For this review, take the finished solid that the model builds, in its own axes (mm). Face numbers are marked on the shaded views. A direction names the side the tool comes from. Round coordinates to 2 decimals unless told otherwise and drop trailing zeros. Order: outer loops, then holes, each group sorted by start corner. A loop starts at its lowest first (then second) coordinate and runs counter-clockwise, first axis right, second up. Notation, with made-up numbers: M 36.5,65 L 85.5,65 A17 ccw 85.5,90 Z; hole C 16.5,7 d2. An arc over 180 degrees is marked long. Write item = value, one per line. Start each with the question number.
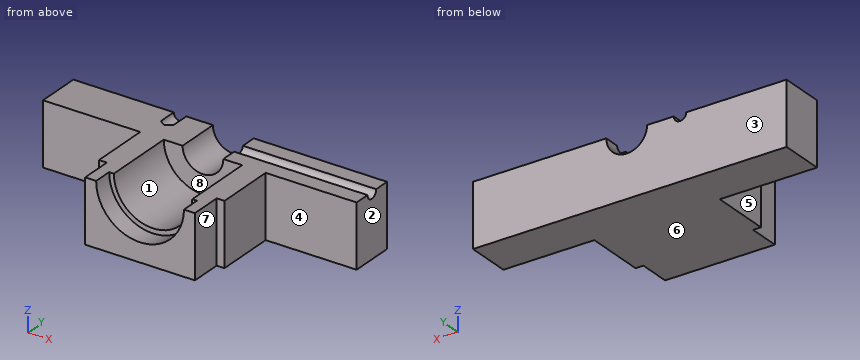
from build123d import *

# Parameters (mm, degrees)
PAD_DEPTH    = 20
SKETCH002_R  = 2
POCKET_DEPTH = 50


with BuildPart() as part:
    # Sketch → Pad (new body)
    with BuildSketch(Plane.XY):
        Polygon((-51, 0), (49, 0), (49, -14), (20, -14), (20, -33), (17.5, -33), (17.5, -43), (-17.5, -43), (-17.5, -33), (-20, -33), (-20, -14), (-51, -14), align=None)
    extrude(amount=-PAD_DEPTH)

    # Sketch001 → Groove (revolve, cut)
    with BuildSketch(Plane.XY):
        Polygon((0, 0), (6.5, 0), (6.5, -14), (12.5, -14), (12.5, -37), (14, -37), (14, -45), (0, -45), align=None)
    revolve(axis=Axis((0, 0, 0), (0, 1, 0)), mode=Mode.SUBTRACT)

    # Sketch002 → Pocket (cut)
    with BuildSketch(Plane.YZ):
        with Locations((-7, 0)):
            Circle(SKETCH002_R)
    extrude(amount=POCKET_DEPTH, mode=Mode.SUBTRACT)

    # Sketch003 → Groove001 (revolve, cut)
    with BuildSketch(Plane(origin=(-17, 0, 0), x_dir=(1, 0, 0), z_dir=(0, 0, 1))):
        Polygon((0, 0), (2, 0), (2, -6), (0, -7.201721), align=None)
    revolve(axis=Axis((-17, 0, 0), (0, 1, 0)), mode=Mode.SUBTRACT)


solid = part.part
(1) For line 1 along Y through (x, z) = (20.5, -4); line 2 along X through (y, z) = (-36.5, -17.5); line 3 along X through (y, z) = (-27, -10), list the stretches that pass through material, from the lowest coordinate up.
(2) Insertion check: pin 1 (8 mm diameter, centred on y = -39.5, z = -14.5, fed in from -X); pin 2 (6 mm diameter, centred on x = 32, z = -9, fed in from -Y); pin 3 (1.2 mm diameter, centred on x = 18.5, z = -5, fed in from -Y). Each pin has a flat end and moves straight along its axis. Give the tip position at first contact, or say it passes through.
(3) We need section B-B, the plane y = -34.5. Write out the cut boundary in (x, z), then the cut area to 3 significant figures.
(4) We need section C-C, the plane z = -15.25. Write out the cut boundary in (x, y).
(5) For the marked faces 1, 2, 3, 4 and 5, list the 3-axis set-ups (+Z, -Z, +X, -X, +Y, -Y) from which the entire face can be reached by the end or side of a thin tool; tool diameter is ignored.
(6) We need section D-D, the plane z = -5.25. Write out the cut boundary in (x, y).
(7) We need section A-A, the plane x = 0. Write out the cut boundary in (y, z), then the cut area to 4 significant figures.
(8) Draft analysis for pull direction X (two halves, no side actions). For the marked faces 6, 7 and 8, state which applies: released by +X, released by -X, zero draft, split by the parting line, or undercut.
Values:
q1.line_1 = -14 to 0
q1.line_2 = -17.5 to 17.5
q1.line_3 = -20 to -7.5, 7.5 to 20
q2.pin_1 = -17.5
q2.pin_2 = -14
q2.pin_3 = -33
q3.outline = M -17.5,-20 L 17.5,-20 L 17.5,0 L 12.5,0 A12.5 cw -12.5,0 L -17.5,0 Z
q3.area = 455 mm²
q4.outline = M -51,-14 L -20,-14 L -20,-33 L -17.5,-33 L -17.5,-43 L 17.5,-43 L 17.5,-33 L 20,-33 L 20,-14 L 49,-14 L 49,0 L -51,0 Z
q5.face_1 = +Z, -Y
q5.face_2 = +Z, -Z, +X, +Y, -Y
q5.face_3 = +Z, -Z, +X, -X, +Y
q5.face_4 = +Z, -Z, +X, -Y
q5.face_5 = +Z, -Z, -X, -Y
q6.outline = M -51,-14 L -20,-14 L -20,-33 L -17.5,-33 L -17.5,-43 L -12.98,-43 L -12.98,-37 L -11.34,-37 L -11.34,-14 L -3.83,-14 L -3.83,0 L -51,0 Z; M 3.83,-14 L 11.34,-14 L 11.34,-37 L 12.98,-37 L 12.98,-43 L 17.5,-43 L 17.5,-33 L 20,-33 L 20,-14 L 49,-14 L 49,0 L 3.83,0 Z
q7.outline = M -43,-20 L 0,-20 L 0,-6.5 L -14,-6.5 L -14,-12.5 L -37,-12.5 L -37,-14 L -43,-14 Z
q7.area = 397.5 mm²
q8.face_6 = zero draft
q8.face_7 = released by +X
q8.face_8 = undercut
